The listing builds one solid part. Answer for the finished solid, in the listing's coordinates (mm). Face numbers are marked on the shaded views. A direction names the side the tool comes from. Give positions to 0.01 mm unless a question says otherwise; leave off trailing zeros. Order: outer loops, then holes, each group sorted by start corner. A loop starts at its lowest first (then second) coordinate and runs counter-clockwise, first axis right, second up. Notation, with made-up numbers: M 8,68 L 52,68 A20 ccw 52,86 Z; hole C 37,-5.5 d3. An arc over 180 degrees is marked long. Answer as a JSON object with one key per item and string values. Group by question number.
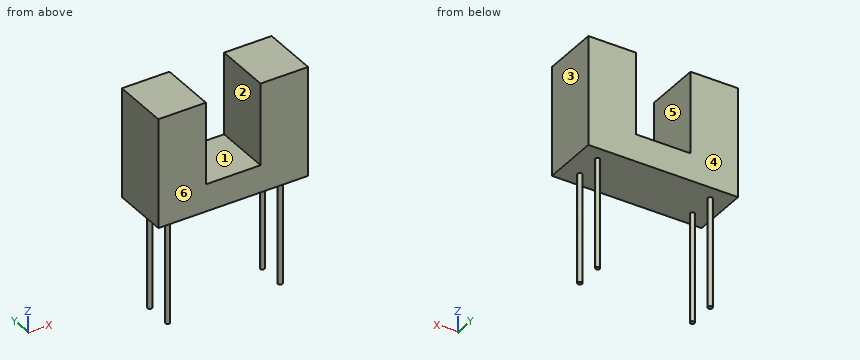
```python
from build123d import *

# Parameters (mm, degrees)
SKETCH1_W           = 13.7
SKETCH1_H           = 10
BOSS_EXTRUDE1_DEPTH = 5.2
SKETCH2_W           = 5
SKETCH2_H           = 7.5
CUT_EXTRUDE1_DEPTH  = 10.947989747
SKETCH3_R           = 0.2
BOSS_EXTRUDE2_DEPTH = 10


with BuildPart() as part:
    # Sketch1 → Boss-Extrude1 (new body)
    with BuildSketch(Plane(origin=(0, 0, 0), x_dir=(1, 0, 0), z_dir=(0, 1, 0))):
        Rectangle(SKETCH1_W, SKETCH1_H)
    extrude(amount=BOSS_EXTRUDE1_DEPTH)

    # Sketch2 → Cut-Extrude1 (cut, through all)
    with BuildSketch(Plane.XZ):
        with Locations((0, 1.25)):
            Rectangle(SKETCH2_W, SKETCH2_H)
    extrude(amount=-CUT_EXTRUDE1_DEPTH, mode=Mode.SUBTRACT)

    # Sketch3 → Boss-Extrude2 (add)
    with BuildSketch(Plane(origin=(0, 0, -5), x_dir=(-1, 0, 0), z_dir=(0, 0, -1))):
        with Locations(Location((-5.15, 3.87, 0), (0, 0, 180))):
            Circle(SKETCH3_R)
        with Locations(Location((-5.15, 1.33, 0), (0, 0, 180))):
            Circle(SKETCH3_R)
        with Locations(Location((5.15, 3.87, 0), (0, 0, 180))):
            Circle(SKETCH3_R)
        with Locations(Location((5.15, 1.33, 0), (0, 0, 180))):
            Circle(SKETCH3_R)
    extrude(amount=BOSS_EXTRUDE2_DEPTH)


solid = part.part
```
Item 1: Determine the mould class of the marked faces 1, 2, 3 and 4 for opening direction X: released by +X, released by -X, zero draft, split by the parting line, or undercut.
Item 2: Section A-A (z = 2.25) is taken. Determine the outline of the cut face in (x, y), and give its area (3 significant figures).
Item 3: A tool of negligible diameter and unlimited length cuts with its end or side. For the marked faces 5 and 6, from which of +Z, -Z, +X, -X, +Y, -Y can it reach the whole face along a straight path? Write none if from no direction.
Item 4: Section D-D (z = -9) is taken. Determine the outline of the cut face in (x, y), and give its area (3 significant figures).
Item 5: Section B-B (x = -5.15) is taken. Determine the outline of the cut face in (y, z), and give its area (3 significant figures).
Item 6: Section C-C (y = 3.87) is taken. Determine the outline of the cut face in (x, z), and give its area (4 significant figures).
Item 7: A flat-ended cylindrical pin translates along its axis: P1, Ø1.5, axis at x = -0.5, y = 3.5, coming from the +Z side. Find the tip coordinate at first contact, or state that the pin passes through.
Item 8: Consider probe 1 along X at (y, z) = (4.7, -2.25); probe 2 along Z at (x, y) = (-0.5, 1.95); probe 3 along Z at (x, y) = (-3.75, 4.4). Determine where each line is inside the solid, lowest interval first. Write a range as from..to.
Values found:
{
 "1": {"face 1": "undercut", "face 2": "undercut", "face 3": "released by +X", "face 4": "zero draft"},
 "2": {"outline": "M -6.85,0 L -2.5,0 L -2.5,5.2 L -6.85,5.2 Z; M 2.5,0 L 6.85,0 L 6.85,5.2 L 2.5,5.2 Z", "area": "45.2 mm^2"},
 "3": {"face 5": "+Z, +Y, -Y", "face 6": "+Z, -Z, +X, -X, -Y"},
 "4": {"outline": "C -5.15,1.33 d0.4; C -5.15,3.87 d0.4; C 5.15,1.33 d0.4; C 5.15,3.87 d0.4", "area": "0.503 mm^2"},
 "5": {"outline": "M 0,-5 L 1.13,-5 L 1.13,-15 L 1.53,-15 L 1.53,-5 L 3.67,-5 L 3.67,-15 L 4.07,-15 L 4.07,-5 L 5.2,-5 L 5.2,5 L 0,5 Z", "area": "60.0 mm^2"},
 "6": {"outline": "M -6.85,-5 L -5.35,-5 L -5.35,-15 L -4.95,-15 L -4.95,-5 L 4.95,-5 L 4.95,-15 L 5.35,-15 L 5.35,-5 L 6.85,-5 L 6.85,5 L 2.5,5 L 2.5,-2.5 L -2.5,-2.5 L -2.5,5 L -6.85,5 Z", "area": "107.5 mm^2"},
 "7": {"P1": "stops at z = -2.5"},
 "8": {"probe 1": "x = -6.85..-2.5, 2.5..6.85", "probe 2": "z = -5..-2.5", "probe 3": "z = -5..5"}
}
